Design review of the part built by this model. Coordinates are the model's own, in mm. A direction names the side the tool comes from. Coordinates: 2 decimals unless noted, no trailing zeros. Order: outer loops, then holes, each group sorted by start corner. A loop starts at its lowest first (then second) coordinate and runs counter-clockwise, first axis right, second up.
Autodesk Inventor part; units mm, degrees
ref_plane "YZ Plane" through (0, 0, 0) normal (1, 0, 0) x (0, 1, 0)
ref_plane "XZ Plane" through (0, 0, 0) normal (0, 1, 0) x (-1, 0, 0)
ref_plane "XY Plane" through (0, 0, 0) normal (0, 0, 1) x (1, 0, 0)
sketch "Sketch1" plane through (0, 0, 0) normal (0, 0, 1) x (1, 0, 0)
  line L0 (-6.25, -7.25) -> (6.25, -7.25)
  line L1 (6.25, -7.25) -> (6.25, 7.25)
  line L2 (6.25, 7.25) -> (-6.25, 7.25)
  line L3 (-6.25, 7.25) -> (-6.25, -7.25)
  line L4 (-6.25, -7.25) -> (6.25, 7.25) construction
  line L5 (6.25, -7.25) -> (-6.25, 7.25) construction
  line L6 (-8.75, -9.75) -> (8.75, -9.75)
  line L7 (8.75, -9.75) -> (8.75, 9.75)
  line L8 (8.75, 9.75) -> (-8.75, 9.75)
  line L9 (-8.75, 9.75) -> (-8.75, -9.75)
  line L10 (-8.75, -9.75) -> (8.75, 9.75) construction
  line L11 (8.75, -9.75) -> (-8.75, 9.75) construction
  line L12 (-3.75, -4.75) -> (3.75, -4.75)
  line L13 (3.75, -4.75) -> (3.75, 4.75)
  line L14 (3.75, 4.75) -> (-3.75, 4.75)
  line L15 (-3.75, 4.75) -> (-3.75, -4.75)
  line L16 (-3.75, -4.75) -> (3.75, 4.75) construction
  line L17 (3.75, -4.75) -> (-3.75, 4.75) construction
  point P0 (0, 0)
  dimension "d0" = 12.5
  dimension "d1" = 14.5
  dimension "d2" = 17.5
  dimension "d3" = 19.5
  dimension "d4" = 7.5
  dimension "d5" = 9.5
extrude "Extrusion1" add sketch "Sketch1" along normal blind 2.5 contours L3 L2 L1 L0 | L9 L8 L7 L6
extrude "Extrusion2" add sketch "Sketch1" against normal blind 7.5 contours L9 L8 L7 L6
properties part number "Adafruit_1528_4663-ND_House_01"
1. Add section D-D (x = 5.5). Give the boundary of the cut face in (y, z).
2. For faces 1 (the flat face through (0, -4.75, 1)), 2 (the flat face through (8.75, 0, -2)), 3 (the flat face through (-4, 0, 0)), list the 3-axis set-ups (+Z, -Z, +X, -X, +Y, -Y) from which the entire face can be reached by the end or side of a thin tool; tool diameter is ignored.
3. Add section B-B (z = -3). Give the boundary of the cut face in (x, y).
4. To check wall thickness, follow line 1 (X direction, y = 1.25, z = -3); line 2 (Y direction, x = -5, z = -5.5); line 3 (Y direction, x = -2.75, z = 0.25). State the ranges of each line that lie inside material, in increasing order.
5. Add section A-A (x = -0.25). Give the boundary of the cut face in (y, z), and give its area (3 significant figures).
6. Add section C-C (y = 3). Give the boundary of the cut face in (x, z).
7. Mouldability with a two-part tool opening along Y and no side actions: class faces 4 (the flat face through (0, -9.75, -2)), 5 (the flat face through (6.25, 0, -4)), 6 (the flat face through (4, 0, 2.5)) as pulls with the +Y half, pulls with the -Y half, needs draft (parallel to the pull), parting line crosses it, or undercut.
Solution:
1. outline: (-9.75, -7.5) - (-7.25, -7.5) - (-7.25, 0) - (7.25, 0) - (7.25, -7.5) - (9.75, -7.5) - (9.75, 2.5) - (-9.75, 2.5) - close
2. face 1: +Z, -Z
2. face 2: +Z, -Z, +X, +Y, -Y
2. face 3: -Z
3. outline: (-8.75, -9.75) - (8.75, -9.75) - (8.75, 9.75) - (-8.75, 9.75) - close; hole (-6.25, -7.25) - (6.25, -7.25) - (6.25, 7.25) - (-6.25, 7.25) - close
4. line 1: x = -8.75 to -6.25, 6.25 to 8.75
4. line 2: y = -9.75 to -7.25, 7.25 to 9.75
4. line 3: y = -9.75 to -4.75, 4.75 to 9.75
5. outline: (-9.75, -7.5) - (-7.25, -7.5) - (-7.25, 0) - (-4.75, 0) - (-4.75, 2.5) - (-9.75, 2.5) - close; (4.75, 0) - (7.25, 0) - (7.25, -7.5) - (9.75, -7.5) - (9.75, 2.5) - (4.75, 2.5) - close
5. area: 62.5 mm2
6. outline: (-8.75, -7.5) - (-6.25, -7.5) - (-6.25, 0) - (-3.75, 0) - (-3.75, 2.5) - (-8.75, 2.5) - close; (3.75, 0) - (6.25, 0) - (6.25, -7.5) - (8.75, -7.5) - (8.75, 2.5) - (3.75, 2.5) - close
7. face 4: pulls with the -Y half
7. face 5: undercut
7. face 6: needs draft
